Design review of the part built by this model. Coordinates are the model's own, in mm. A direction names the side the tool comes from. Round coordinates to 2 decimals unless told otherwise and drop trailing zeros. Loops run counter-clockwise (first coordinate to the right, second up) from the corner with the lowest first, then second, coordinate; pieces in that order, holes last. Notation, with made-up numbers: (43.5, 28) - (83.5, 28) arc R29 ccw to (83.5, 59) - close; hole circle Ø11 at (85, 64). An arc over 180 degrees is marked (long way). Return JSON: item names as keys, results as strings. Group by question number.
(1) Clearance check with flat-ended pins moving along their axes: pin 1 (18 mm diameter, centred on x = 101.5, z = -0.5, fed in from +Y); pin 2 (5 mm diameter, centred on x = 77, y = 35.5, fed in from +Z); pin 3 (3 mm diameter, centred on x = 98, y = 35.5, fed in from -Z). State where each tip first meets the part, or that it passes through.
(2) We need section D-D, the plane x = 74. Write out the cut boundary in (y, z).
(3) We need section A-A, the plane z = 0. Write out the cut boundary in (x, y), and give its area (3 significant figures).
(4) Wall thickness on L1, parallel to Z at x = 74, y = 19.5; L2, parallel to X at y = 4.5, z = 54; L3, parallel to Z at x = 83.5, y = 16: over which ranges is each line inside the solid? List them lowest first. Write a range as [from, to].
(5) The part is to be moulded in two halves that separate along Z. For faces 1 (the flat face through (15.8, 92.8, 87.4)), 2 (the cylindrical face through (58, 7, -42)), 3 (the flat face through (46, 16, -100)), 4 (the flat face through (0, 86, 21)), say which applies: pulls with the +Z half, pulls with the -Z half, needs draft (parallel to the pull), parting line crosses it, or undercut.
(6) We need section B-B, the plane x = 25. Write out the cut boundary in (y, z), and give its area (3 significant figures).
(7) For faces 5 (the flat face through (90, 32, -78)), 6 (the flat face through (74, 2, -54)), 7 (the flat face through (79, 37, 18)), list the 3-axis set-ups (+Z, -Z, +X, -X, +Y, -Y) from which the entire face can be reached by the end or side of a thin tool; tool diameter is ignored.
(8) We need section C-C, the plane y = 27. Write out the cut boundary in (x, z).
from build123d import *

# Parameters (mm, degrees)
BOSS_EXTRUDE1_DEPTH   = 32
BOSS_EXTRUDE1_2_DEPTH = 32
SKETCH1_3_W           = 128
SKETCH1_3_H           = 18
BOSS_EXTRUDE2_DEPTH   = 42
SKETCH2_R             = 22.5
BOSS_EXTRUDE3_DEPTH   = 32
SKETCH4_R             = 20
SKETCH4_R_2           = 26
CUT_EXTRUDE1_DEPTH    = 20
SKETCH4_3_R           = 20
CUT_EXTRUDE2_DEPTH    = 30


with BuildPart() as part:
    # Sketch1 → Boss-Extrude1 (new body)
    with BuildSketch(Plane(origin=(0, 0, 0), x_dir=(1, 0, 0), z_dir=(0, 1, 0))):
        Polygon((0, -18), (0, -100), (90, -100), (128, -62), (128, -18), align=None)
    extrude(amount=BOSS_EXTRUDE1_DEPTH)



with BuildPart() as body_2:
    # Sketch1 → Boss-Extrude1 2 (new body)
    with BuildSketch(Plane(origin=(0, 0, 0), x_dir=(1, 0, 0), z_dir=(0, 1, 0))):
        Polygon((0, 100), (0, 18), (128, 18), (128, 62), (90, 100), align=None)
    extrude(amount=BOSS_EXTRUDE1_2_DEPTH)


with BuildPart() as part_1:
    add(part.part)

    add(body_2.part)  # Boss-Extrude2 merges body 2
    # Sketch1_3 → Boss-Extrude2 (add)
    with BuildSketch(Plane(origin=(0, 0, 0), x_dir=(1, 0, 0), z_dir=(0, 1, 0))):
        with Locations((64, 9)):
            Rectangle(SKETCH1_3_W, SKETCH1_3_H)
        with Locations((64, -9)):
            Rectangle(SKETCH1_3_W, SKETCH1_3_H)
    extrude(amount=BOSS_EXTRUDE2_DEPTH)

    # Sketch2 → Boss-Extrude3 (add)
    with BuildSketch(Plane(origin=(0, 0, 0), x_dir=(0, 0, -1), z_dir=(1, 0, 0))):
        with BuildLine():
            Line((-100, 32), (-74.418333794, 155.424383143))
            ThreePointArc((-74.418333794, 155.424383143), (0, 216), (74.418333794, 155.424383143))
            Line((74.418333794, 155.424383143), (100, 32))
            Line((100, 32), (-100, 32))
        make_face()
        with Locations((0, 96)):
            Circle(SKETCH2_R, mode=Mode.SUBTRACT)
    extrude(amount=BOSS_EXTRUDE3_DEPTH)

    # Sketch4 → Cut-Extrude1 (cut)
    with BuildSketch(Plane(origin=(0, 32, 0), x_dir=(1, 0, 0), z_dir=(0, 1, 0))):
        with Locations((74, 54)):
            Circle(SKETCH4_R)
        with Locations((74, 54)):
            Circle(SKETCH4_R_2)
        with Locations((74, 54)):
            Circle(SKETCH4_R, mode=Mode.SUBTRACT)
        with Locations((74, -54)):
            Circle(SKETCH4_R_2)
        with Locations((74, -54)):
            Circle(SKETCH4_R, mode=Mode.SUBTRACT)
        with Locations((74, -54)):
            Circle(SKETCH4_R)
    extrude(amount=-CUT_EXTRUDE1_DEPTH, mode=Mode.SUBTRACT)

    # Sketch4_3 → Cut-Extrude2 (cut)
    with BuildSketch(Plane(origin=(0, 32, 0), x_dir=(1, 0, 0), z_dir=(0, 1, 0))):
        with Locations((74, 54)):
            Circle(SKETCH4_3_R)
        with Locations((74, -54)):
            Circle(SKETCH4_3_R)
    extrude(amount=-CUT_EXTRUDE2_DEPTH, mode=Mode.SUBTRACT)


solid = part_1.part
Solutions:
{
 "1": {"pin 1": "y = 42", "pin 2": "z = 18", "pin 3": "z = -18"},
 "2": {"outline": "(0, -100) - (32, -100) - (32, -80) - (12, -80) - (12, -74) - (2, -74) - (2, -34) - (12, -34) - (12, -28) - (32, -28) - (32, -18) - (42, -18) - (42, 18) - (32, 18) - (32, 28) - (12, 28) - (12, 34) - (2, 34) - (2, 74) - (12, 74) - (12, 80) - (32, 80) - (32, 100) - (0, 100) - close"},
 "3": {"outline": "(0, 0) - (128, 0) - (128, 42) - (32, 42) - (32, 73.5) - (0, 73.5) - close; (0, 118.5) - (32, 118.5) - (32, 216) - (0, 216) - close", "area": "9,500 mm^2"},
 "4": {"L1": "[-100, -80], [-28, 28], [80, 100]", "L2": "[0, 54], [94, 128]", "L3": "[-100, -78.2], [-29.8, 29.8], [78.2, 100]"},
 "5": {"face 1": "pulls with the +Z half", "face 2": "undercut", "face 3": "pulls with the -Z half", "face 4": "needs draft"},
 "6": {"outline": "(0, -100) - (32, -100) - (155.42, -74.42) arc R76 ccw to (155.42, 74.42) - (32, 100) - (0, 100) - close; hole circle Ø45 at (96, 0)", "area": "33,100 mm^2"},
 "7": {"face 5": "-Z, +X, +Y", "face 6": "+Y", "face 7": "+Z, +X, +Y"},
 "8": {"outline": "(0, -100) - (90, -100) - (128, -62) - (128, 62) - (90, 100) - (0, 100) - close; hole circle Ø52 at (74, -54); hole circle Ø52 at (74, 54)"}
}
